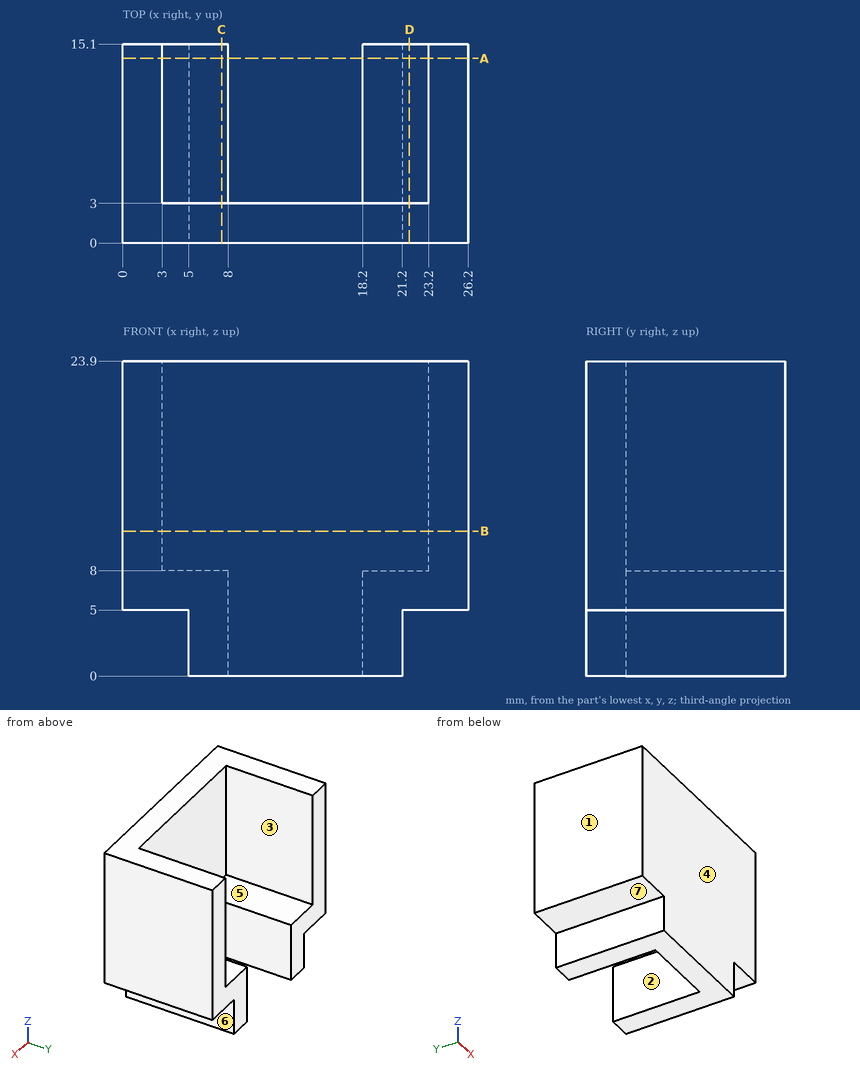
Answer from the drawing. Dimensions are ordinates in mm from the lowest x, y and z of the part. A direction names the side the tool comes from. Coordinates: 2 decimals unless noted, no trailing zeros. Write each loop counter-clockwise with the first axis right and the second up, starting at its lowest first coordinate (ties: lowest second). Pieces come first, ordered by that corner, then holes. Notation, with made-up numbers: (3, 50) - (47, 50) arc R17 ccw to (47, 64) - close; hole circle Ø9 at (87.25, 76.25). An arc over 180 degrees is marked (long way). Return JSON: item names as keys, results as strings.
1. For a pull along X with two mould halves and no side action, classify the marked faces 1, 2, 3 and 4 as +X half, -X half, draft (parallel to the pull), parting line (faces both ways), or undercut.
Final values:
{"face 1": "-X half", "face 2": "undercut", "face 3": "undercut", "face 4": "draft"}
2. Each of these flat-tipped pins is pushed along its axis until it touches: pin 1 Ø4 at (y, z) = (1.5, 11.5) entering from -X; pin 2 Ø12 at (x, z) = (14, 13.5) entering from +Y; pin 3 Ø4 at (y, z) = (9.5, 2.5) entering from +X; pin 4 Ø2.5 at (x, y) = (21.5, 10) entering from +Z. Where does it stop, or does it pass through?
Final values:
{"pin 1": "x = 0", "pin 2": "y = 3", "pin 3": "x = 21.2", "pin 4": "z = 8"}
3. Consider line 1 along X through (y, z) = (11.5, 1); line 2 along X through (y, z) = (6.5, 14.25); line 3 along Z through (x, y) = (22.25, 12.25). Determine where each line is inside the solid, lowest interval first.
Final values:
{"line 1": "5 to 8, 18.2 to 21.2", "line 2": "0 to 3, 23.2 to 26.2", "line 3": "5 to 8"}
4. Which of the six approach directions +Z, -Z, +X, -X, +Y, -Y give full straight-line access (tool end or side, diameter ignored) to the marked faces 5, 6 and 7?
Final values:
{"face 5": "+Z, +Y", "face 6": "-Z, +X, +Y, -Y", "face 7": "-Z, -X, +Y, -Y"}
5. The part is cut by section C-C on x = 7.5. Determine the outline of the cut face in (y, z).
Final values:
{"outline": "(0, 0) - (15.1, 0) - (15.1, 8) - (3, 8) - (3, 23.9) - (0, 23.9) - close"}
6. The part is cut by section D-D on x = 21.75. Determine the outline of the cut face in (y, z).
Final values:
{"outline": "(0, 5) - (15.1, 5) - (15.1, 8) - (3, 8) - (3, 23.9) - (0, 23.9) - close"}
7. The part is cut by section A-A on y = 14. Determine the outline of the cut face in (x, z).
Final values:
{"outline": "(0, 5) - (5, 5) - (5, 0) - (8, 0) - (8, 8) - (3, 8) - (3, 23.9) - (0, 23.9) - close; (18.2, 0) - (21.2, 0) - (21.2, 5) - (26.2, 5) - (26.2, 23.9) - (23.2, 23.9) - (23.2, 8) - (18.2, 8) - close"}
8. The part is cut by section B-B on z = 11. Determine the outline of the cut face in (x, y).
Final values:
{"outline": "(0, 0) - (26.2, 0) - (26.2, 15.1) - (23.2, 15.1) - (23.2, 3) - (3, 3) - (3, 15.1) - (0, 15.1) - close"}
